The listing builds one solid part. Answer for the finished solid, in the listing's coordinates (mm). A direction names the side the tool comes from. Round coordinates to 2 decimals unless told otherwise and drop trailing zeros. Loops run counter-clockwise (first coordinate to the right, second up) from the corner with the lowest first, then second, coordinate; pieces in that order, holes last. Notation, with made-up numbers: (82.5, 62) - (134.5, 62) arc R31 ccw to (134.5, 101) - close; hole circle Ø7 at (49.5, -4.5). An arc over 180 degrees is marked (long way). Write item = value, one per line. Start each with the question number.
1) Section C-C, the plane x = 15.5 is taken. Determine the outline of the cut face in (y, z), and give its area (3 significant figures).
2) Section A-A, the plane y = -15 is taken. Determine the outline of the cut face in (x, z), and give its area (3 significant figures).
3) Section D-D, the plane y = -26.5 is taken. Determine the outline of the cut face in (x, z), and give its area (3 significant figures).
4) For a pull along Y with two mould halves and no side action, classify faces 1 (the flat face through (10, -4, 2)), 2 (the cylindrical face through (22.288, -0.958, 2.594)), 3 (the flat face through (15, -24, 3)) as released by +Y, released by -Y, zero draft, split by the parting line, or undercut.
5) Section B-B, the plane z = 5.6 is taken. Determine the outline of the cut face in (x, y), and give its area (3 significant figures).
6) Given pin 1 Ø1.6 at (x, z) = (10, 3) entering from +Y, flat-ended and moving along its own axis, determine where the tip first touches the part or whether it passes through.
7) A tool of negligible diameter and unlimited length cuts with its end or side. For faces 4 (the cylindrical face through (11.247, -0.958, 3.517)), 5 (the flat face through (15, 2, 1)), 6 (the flat face through (22.883, -5, 5)), 7 (the flat face through (15, -26, 2)), 8 (the flat face through (4.5, -15, 3)), from which of +Z, -Z, +X, -X, +Y, -Y can it reach the whole face along a straight path? Write none if from no direction.
8) Straight lines are drawn through the part: line 1 along Y through (x, z) = (8.5, 3.1); line 2 along X through (y, z) = (-30.7, 3); line 3 along Z through (x, y) = (21, 0). For each, find the intervals that lie inside material, in ascending order.
Autodesk Inventor part; units mm, degrees
ref_plane "YZ Plane" through (0, 0, 0) normal (1, 0, 0) x (0, 1, 0)
ref_plane "XZ Plane" through (0, 0, 0) normal (0, 1, 0) x (-1, 0, 0)
ref_plane "XY Plane" through (0, 0, 0) normal (0, 0, 1) x (1, 0, 0)
sketch "스케치1" plane through (0, 0, 0) normal (0, 0, 1) x (1, 0, 0)
  line L0 (28.5, 0) -> (46.5, 0)
  line L1 (46.5, 0) -> (46.5, -1.5)
  line L2 (50.5, -1.5) -> (46.5, -1.5)
  line L3 (50.5, 0) -> (50.5, -1.5)
  line L4 (50.5, 0) -> (53.1, 0)
  line L5 (53.1, 0) -> (53.1, 2)
  line L6 (0, 2) -> (53.1, 2)
  line L7 (0, 0) -> (0, 2)
  line L8 (0, 0) -> (2.5, 0)
  line L9 (2.5, 0) -> (2.5, -1.5)
  line L10 (6.5, -1.5) -> (2.5, -1.5)
  line L11 (6.5, 0) -> (6.5, -1.5)
  line L12 (6.5, 0) -> (24.5, 0)
  line L13 (24.5, 0) -> (24.5, -1.5)
  line L14 (28.5, -1.5) -> (24.5, -1.5)
  line L15 (28.5, 0) -> (28.5, -1.5)
  line L16 (8.475, -27.5) -> (6.975, -27.5)
  line L17 (6.975, -27.5) -> (6.975, -29.5)
  line L18 (6.975, -29.5) -> (2.025, -29.5)
  line L19 (2.025, -27.5) -> (2.025, -29.5)
  line L20 (2.025, -27.5) -> (0.525, -27.5)
  line L21 (0.525, -27.5) -> (0.525, -30)
  line L22 (0, -30) -> (0.525, -30)
  line L23 (0, -30) -> (0, -32)
  line L24 (0, -32) -> (53.1, -32)
  line L25 (53.1, -30) -> (53.1, -32)
  line L26 (52.475, -30) -> (53.1, -30)
  line L27 (52.475, -30) -> (52.475, -27.5)
  line L28 (52.475, -27.5) -> (50.975, -27.5)
  line L29 (50.975, -27.5) -> (50.975, -29.5)
  line L30 (50.975, -29.5) -> (46.025, -29.5)
  line L31 (46.025, -27.5) -> (46.025, -29.5)
  line L32 (46.025, -27.5) -> (44.525, -27.5)
  line L33 (44.525, -27.5) -> (44.525, -30)
  line L34 (30.475, -30) -> (44.525, -30)
  line L35 (30.475, -30) -> (30.475, -27.5)
  line L36 (30.475, -27.5) -> (28.975, -27.5)
  line L37 (28.975, -27.5) -> (28.975, -29.5)
  line L38 (28.975, -29.5) -> (24.025, -29.5)
  line L39 (24.025, -27.5) -> (24.025, -29.5)
  line L40 (24.025, -27.5) -> (22.525, -27.5)
  line L41 (22.525, -27.5) -> (22.525, -30)
  line L42 (8.475, -30) -> (22.525, -30)
  line L43 (8.475, -30) -> (8.475, -27.5)
  line L44 (48.1766, 5.1) -> (3.9234, 5.1)
  line L45 (29.3, 2) -> (29.3, 8)
  line L46 (3.15, 8) -> (3.15, 2)
  line L47 (1.7, -38) -> (1.7, -32)
  line L48 (29.3, -38) -> (29.3, -32)
  line L49 (15.5, 2) -> (15.5, -15)
  circle A0 centre (8.5, -15) radius 1.5
  line L50 (26.55, 2) -> (26.55, -32)
  line L51 (4.5, 2) -> (4.5, -32)
  dimension "d0" = 17
extrude "돌출1" add sketch "스케치1" along normal blind 6 contours L50 L38 L39 L40 L41 L42 L43 L16 L17 L18 L51 L10 L11 L12 L13 L14 | L14 L13 L12 L49 L6 L50 | L50 L24 L51 L18 L17 L16 L43 L42 L41 L40 L39 L38 | L49 L12 L11 L10 L51 L6
sketch "스케치2" plane through (4.5, 2, 0) normal (0, 1, 0) x (1, 0, 0)
  arc A0 (22, 0) -> (22, 5.6) centre (22, 2.8) ccw
  line L0 (22, 5.6) -> (0, 5.6)
  arc A1 (0, 5.6) -> (0, 0) centre (0, 2.8) ccw
  line L1 (0, 0) -> (0, -6)
  line L2 (0, -6) -> (22, -6)
  line L3 (22, -6) -> (22, 0)
  circle A2 centre (11, -3) radius 1.35
  circle A3 centre (16.5, -3) radius 1.35
  circle A4 centre (0, 2.8) radius 1.35
  circle A5 centre (22, 2.8) radius 1.35
  circle A6 centre (5.5, -3) radius 1.35
  point P0 (-4.5, 0)
extrude "돌출2" cut sketch "스케치2" against normal blind 6 contours A2 | A3 | A6
sketch "스케치3" plane through (4.5, -32, 0) normal (0, -1, 0) x (1, 0, 0)
  arc A0 (22, -5.6) -> (22, 0) centre (22, -2.8) ccw
  line L0 (22, 6) -> (22, 0)
  line L1 (0, 6) -> (22, 6)
  line L2 (0, 0) -> (0, 6)
  arc A1 (0, 0) -> (0, -5.6) centre (0, -2.8) ccw
  line L3 (22, -5.6) -> (0, -5.6)
  circle A2 centre (11, 3) radius 1.35
  circle A3 centre (16.5, 3) radius 1.35
  circle A4 centre (0, -2.8) radius 1.35
  circle A5 centre (22, -2.8) radius 1.35
  circle A6 centre (5.5, 3) radius 1.35
  point P0 (-4.5, 0)
extrude "돌출3" cut sketch "스케치3" against normal blind 6 contours A2 | A3 | A6
sketch "스케치4" plane through (0, 0, 6) normal (0, 0, 1) x (1, 0, 0)
  line L0 (19.65, -4) -> (22.35, -4)
  line L1 (14.15, -4) -> (16.85, -4)
  line L2 (8.65, -4) -> (11.35, -4)
  line L3 (22.35, -26) -> (19.65, -26)
  line L4 (16.85, -26) -> (14.15, -26)
  line L5 (11.35, -26) -> (8.65, -26)
  line L6 (22.883, -4) -> (22.883, -7)
  line L7 (22.883, -7) -> (7.8508, -7)
  line L8 (7.8508, -7) -> (7.8508, -4)
  line L9 (7.8508, -4) -> (22.883, -4)
  line L10 (22.883, -23) -> (22.883, -26)
  line L11 (22.883, -26) -> (7.788, -26)
  line L12 (7.788, -26) -> (7.788, -23)
  line L13 (7.788, -23) -> (22.883, -23)
  line L14 (8.65, -32) -> (8.65, -26)
  line L15 (8.65, 2) -> (8.65, -4)
  point P0 (0, 0)
  dimension "d7" = 3
  dimension "d8" = 3
extrude "돌출4" cut sketch "스케치4" against normal blind 3
properties part number "_adle_adt_2"
Geometry check:
q1.outline = (-32, 0) - (2, 0) - (2, 1.65) - (-4, 1.65) - (-4, 3) - (-7, 3) - (-7, 6) - (-23, 6) - (-23, 3) - (-26, 3) - (-26, 1.65) - (-32, 1.65) - close; (-32, 4.35) - (-26, 4.35) - (-26, 6) - (-32, 6) - close; (-4, 4.35) - (2, 4.35) - (2, 6) - (-4, 6) - close
q1.area = 154 mm2
q2.outline = (4.5, 0) - (7, 0) - (7, 6) - (4.5, 6) - close; (10, 0) - (26.55, 0) - (26.55, 6) - (10, 6) - close
q2.area = 114 mm2
q3.outline = (4.5, 0) - (26.55, 0) - (26.55, 6) - (4.5, 6) - close; hole circle Ø2.7 at (10, 3); hole circle Ø2.7 at (15.5, 3); hole circle Ø2.7 at (21, 3)
q3.area = 115 mm2
q4.face_1 = released by +Y
q4.face_2 = zero draft
q4.face_3 = undercut
q5.outline = (4.5, -32) - (26.55, -32) - (26.55, 2) - (4.5, 2) - close; hole circle Ø3 at (8.5, -15); hole (7.79, -26) - (22.88, -26) - (22.88, -23) - (7.79, -23) - close; hole (7.85, -7) - (22.88, -7) - (22.88, -4) - (7.85, -4) - close
q5.area = 652 mm2
q6.pin_1 = -4
q7.face_4 = +Y
q7.face_5 = +Z, -Z, +X, -X, +Y
q7.face_6 = +Z
q7.face_7 = -Y
q7.face_8 = +Z, -Z, -X, +Y, -Y
q8.line_1 = -32 to -26, -23 to -16.5, -13.5 to -7, -4 to 2
q8.line_2 = 4.5 to 8.65, 11.35 to 14.15, 16.85 to 19.65, 22.35 to 26.55
q8.line_3 = 0 to 1.65, 4.35 to 6
